Print and shaded views of the part. All mm, measured from the part's lowest x, y and z. A direction names the side the tool comes from. Round coordinates to 2 decimals unless told otherwise and drop trailing zeros. Write each loop counter-clockwise with the first axis right and the second up, starting at its lowest first coordinate (ties: lowest second). Pieces come first, ordered by that corner, then holes. Notation, with made-up numbers: (79, 42.25) - (114, 42.25) arc R14 ccw to (114, 59.25) - close; hole circle Ø7 at (-11, 48). An arc over 180 degrees is marked (long way). Put each result on its own line as item: value. Start each with the question number.
Item 1: 3-axis set-ups, long thin cutter, end or side, ignore diameter. For the marked faces 1, 2 and 3: which of +Z, -Z, +X, -X, +Y, -Y reach the whole face in a straight line?
Item 2: Drill centre lines: line 1 (X direction, y = 19.5, z = 11); line 2 (Y direction, x = 17, z = 19.05) (1 decimal); line 3 (Y direction, x = 5.25, z = 19.05) (1 decimal). Where is each one in solid material? Low to high. Write a range as from..to.
Item 3: Cut at A-A (z = 19.05). Count the separate pieces of the cut face and the enclosed holes in it.
Item 4: Pin check, flat tips, straight feed: pin 1 Ø1.5 at (x, z) = (17, 22.5) entering from -Y; pin 2 Ø4 at (x, z) = (2, 25) entering from -Y; pin 3 Ø6.5 at (y, z) = (15.87, 19.05) entering from +X; pin 4 Ø8 at (y, z) = (23.5, 7.5) entering from +X. Stop position of each tip, or through.
Item 5: Cut at B-B (y = 56.5). Give the cut face in (x, z) (1 decimal).
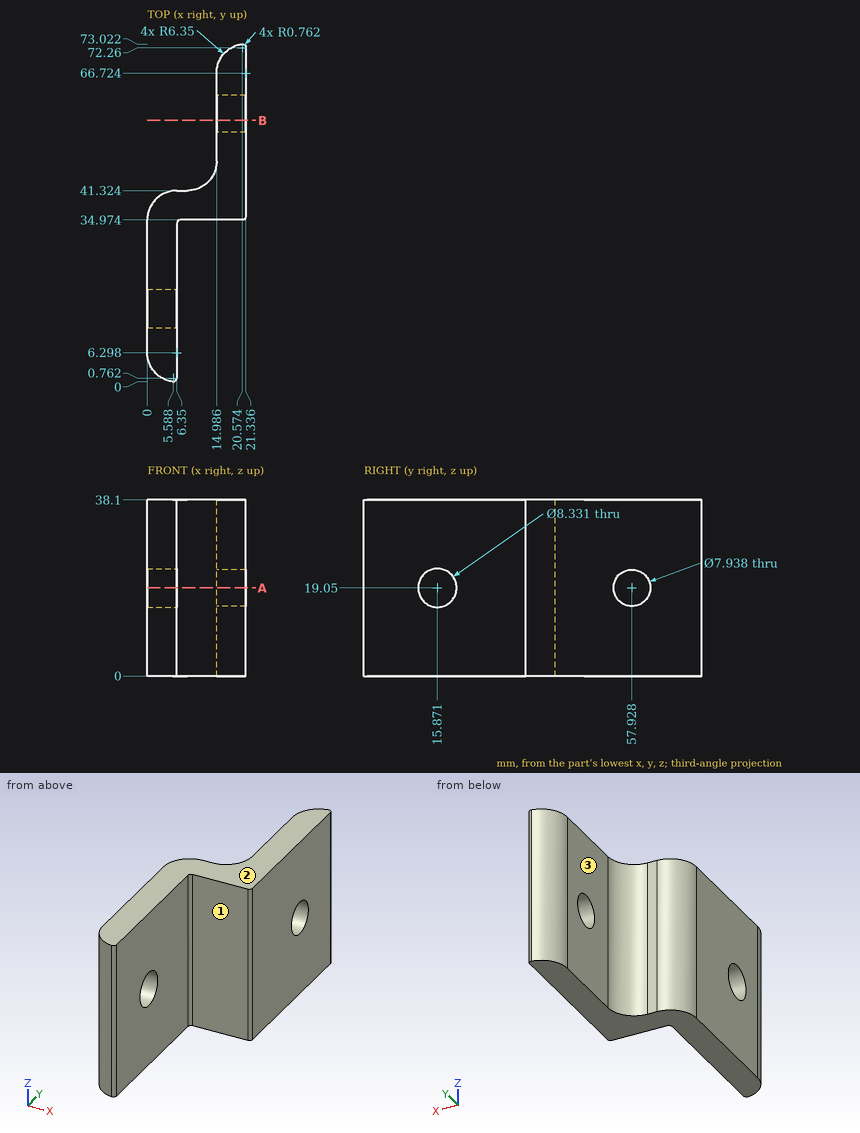
Output values:
1. face 1: +Z, -Z, +X, -Y
1. face 2: +Z, +X, -X, +Y, -Y
1. face 3: +Z, -Z, -X, +Y
2. line 1: 0..6.35
2. line 2: 35..54, 61.9..71.4
2. line 3: 0..11.7, 20..41.2
3. separate pieces: 3
3. enclosed holes: 0
4. pin 1: y = 34.97
4. pin 2: y = 0.4
4. pin 3: through
4. pin 4: x = 6.35
5. outline: (15, 0) - (21.3, 0) - (21.3, 15.3) - (15, 15.3) - close; (15, 22.8) - (21.3, 22.8) - (21.3, 38.1) - (15, 38.1) - close
